Check sheet for the drawn part. Datum: minimum x, y, z corner. Units: mm. Round coordinates to 2 decimals unless told otherwise and drop trailing zeros. Order: outer loops, then holes, each group sorted by start corner. A loop starts at its lowest first (then second) coordinate and runs counter-clockwise, first axis right, second up. Notation, with made-up numbers: (48.5, 47) -> (77.5, 47) arc R25 cw to (77.5, 70) -> close; hole circle Ø4 at (51, 24). An arc over 180 degrees is marked (long way). Answer in a Markdown table with one row per item.
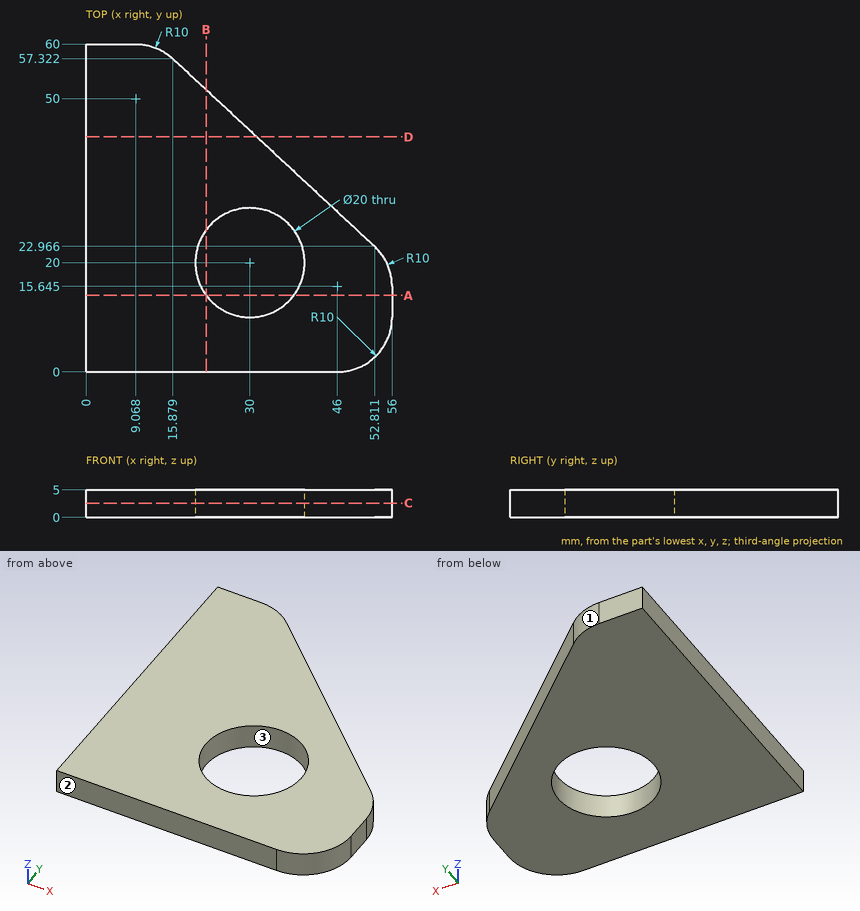
(1) Section check B-B on x = 22. Record the boundary of the cut face in (y, z).
Solutions:
| item | result |
|---|---|
| outline | (0, 0) -> (14, 0) -> (14, 5) -> (0, 5) -> close; (26, 0) -> (51.63, 0) -> (51.63, 5) -> (26, 5) -> close |
(2) Draft check along Y on the marked faces 1, 2 and 3. Enter one of: pulls with the +Y half, pulls with the -Y half, needs draft (parallel to the pull), parting line crosses it, or undercut.
Solutions:
| item | result |
|---|---|
| face 1 | pulls with the +Y half |
| face 2 | pulls with the -Y half |
| face 3 | undercut |
(3) Section check C-C on z = 2.6. Record the boundary of the cut face in (x, y) (1 decimal), plus the area to 3 significant figures.
Solutions:
| item | result |
|---|---|
| outline | (0, 0) -> (46, 0) arc R10 ccw to (56, 10) -> (56, 15.6) arc R10 ccw to (52.8, 23) -> (15.9, 57.3) arc R10 ccw to (9.1, 60) -> (0, 60) -> close; hole circle Ø20 at (30, 20) |
| area | 2,160 mm^2 |
(4) Depth check by flat-ended pin: pin 1 Ø1.5 at (y, z) = (41, 1.5) entering from +X; pin 2 Ø1 at (y, z) = (48.5, 4) entering from -X. Enter the tip coordinate at first touch or a pass-through.
Solutions:
| item | result |
|---|---|
| pin 1 | x = 34.23 |
| pin 2 | x = 0 |
(5) Section check D-D on y = 43. Record the boundary of the cut face in (x, z) (1 decimal).
Solutions:
| item | result |
|---|---|
| outline | (0, 0) -> (31.3, 0) -> (31.3, 5) -> (0, 5) -> close |
(6) Scan lines: probe 1 along Y at (x, z) = (21.5, 3.95) (1 decimal); probe 2 along Y at (x, z) = (26.5, 1.65) (1 decimal); probe 3 along X at (y, z) = (22.5, 3.75) (1 decimal). Record each from-to range of solid material in increasing order. Write a range as from..to.
Solutions:
| item | result |
|---|---|
| probe 1 | 0..14.7, 25.3..52.1 |
| probe 2 | 0..10.6, 29.4..47.4 |
| probe 3 | 0..20.3, 39.7..53.3 |
(7) Section check A-A on y = 14. Record the boundary of the cut face in (x, z).
Solutions:
| item | result |
|---|---|
| outline | (0, 0) -> (22, 0) -> (22, 5) -> (0, 5) -> close; (38, 0) -> (56, 0) -> (56, 5) -> (38, 5) -> close |
